Drawing for the job (mm, zero at the part's lowest x, y, z). A direction names the side the tool comes from. Round coordinates to 2 decimals unless told otherwise and drop trailing zeros. Write each loop counter-clockwise with the first axis right and the second up, starting at its lowest first coordinate (ties: lowest second). Pieces come first, ordered by that corner, then holes. Notation, with made-up numbers: (-27.75, 54) -> (17.25, 54) arc R29 ccw to (17.25, 82) -> close; hole circle Ø6 at (24.5, 87). An arc over 180 degrees is marked (long way). One line per question, with ' | ' between items.
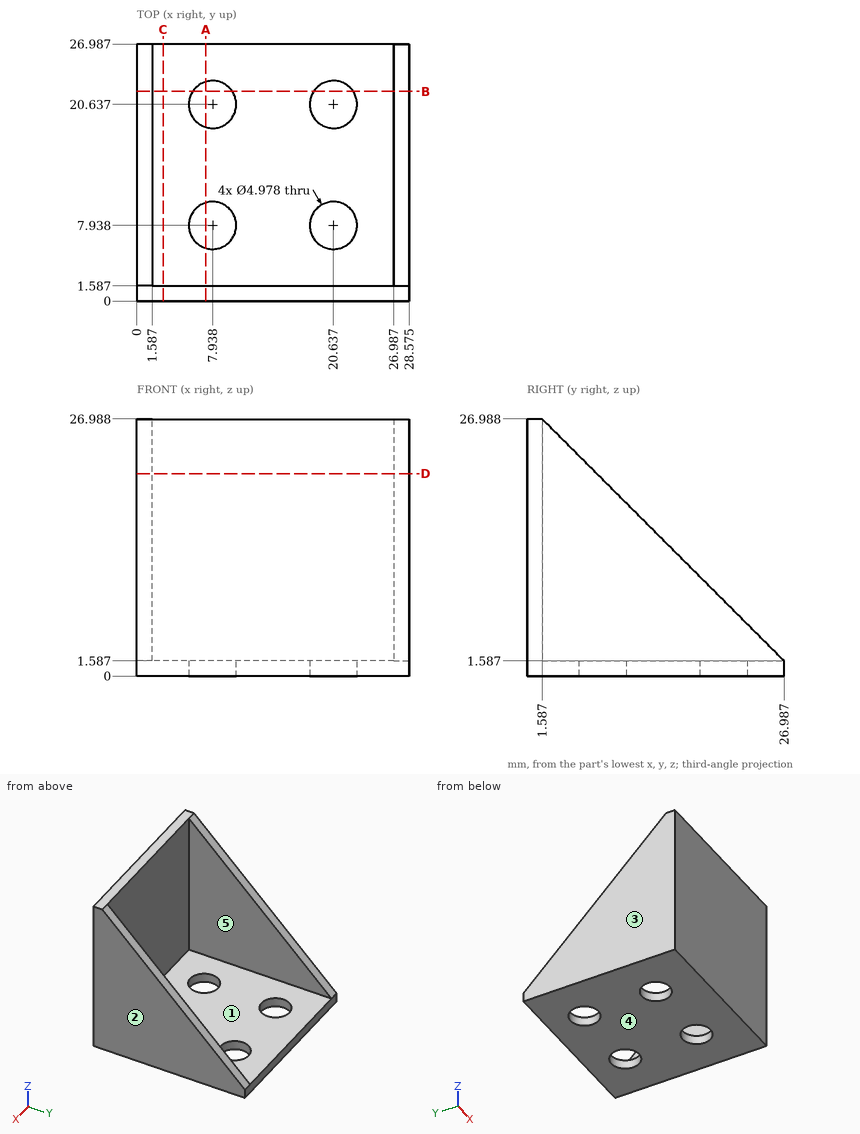
(1) Slice it at D-D (z = 21.25). Write the cut outline in (x, y) (1 decimal).
Calculated:
outline: (0, 0) -> (28.6, 0) -> (28.6, 7.3) -> (27, 7.3) -> (27, 1.6) -> (1.6, 1.6) -> (1.6, 7.3) -> (0, 7.3) -> close
(2) Slice it at A-A (x = 7.25). Write the cut outline in (y, z) (1 decimal).
Calculated:
outline: (0, 0) -> (5.5, 0) -> (5.5, 1.6) -> (1.6, 1.6) -> (1.6, 27) -> (0, 27) -> close; (10.3, 0) -> (18.2, 0) -> (18.2, 1.6) -> (10.3, 1.6) -> close; (23, 0) -> (27, 0) -> (27, 1.6) -> (23, 1.6) -> close
(3) Wall check: line 1 (X direction, y = 25.75, z = 2.5) (1 decimal); line 2 (Y direction, x = 3, z = 13.25). Give the ranges that are in metal, low to high. Write a range as from..to.
Calculated:
line 1: 0..1.6, 27..28.6 | line 2: 0..1.59
(4) Slice it at C-C (x = 2.75). Write the cut outline in (y, z).
Calculated:
outline: (0, 0) -> (26.99, 0) -> (26.99, 1.59) -> (1.59, 1.59) -> (1.59, 26.99) -> (0, 26.99) -> close
(5) Slice it at B-B (y = 22). Write the cut outline in (x, z) (1 decimal).
Calculated:
outline: (0, 0) -> (5.9, 0) -> (5.9, 1.6) -> (1.6, 1.6) -> (1.6, 6.6) -> (0, 6.6) -> close; (10, 0) -> (18.6, 0) -> (18.6, 1.6) -> (10, 1.6) -> close; (22.7, 0) -> (28.6, 0) -> (28.6, 6.6) -> (27, 6.6) -> (27, 1.6) -> (22.7, 1.6) -> close
(6) Drop flat-ended pins along their axis: pin 1 (10 mm diameter, centred on x = 10.5, y = 10, fed in from +Z); pin 2 (8 mm diameter, centred on x = 20.5, z = 21, fed in from +Y); pin 3 (4.5 mm diameter, centred on x = 7.94, y = 7.94, fed in from +Z). Give the stop position or say it passes through.
Calculated:
pin 1: z = 1.59 | pin 2: y = 1.59 | pin 3: through
(7) Mould opens along X. For the marked faces 3, 4 and 5 say: pulls with the +X half, pulls with the -X half, needs draft (parallel to the pull), parting line crosses it, or undercut.
Calculated:
face 3: pulls with the -X half | face 4: needs draft | face 5: undercut
(8) 3-axis set-ups, long thin cutter, end or side, ignore diameter. For the marked faces 1 and 2: which of +Z, -Z, +X, -X, +Y, -Y reach the whole face in a straight line?
Calculated:
face 1: +Z, +Y | face 2: +Z, -Z, +X, +Y, -Y
